```python
from build123d import *

# Parameters (mm, degrees)
F0_W     = 914.4
F0_H     = 914.4
F0_W_2   = 80
F0_H_2   = 40
F1_DEPTH = 40
F2_DEPTH = 1000
F4_W     = 674.4
F4_H     = 40
F5_DEPTH = 127
F7_W     = 674.4
F7_H     = 128
F8_DEPTH = 37
F9_DEPTH = 40


# Not quite as in the source:
# - a feature names something its author has since deleted; it is built from what else it names


with BuildPart() as f1:
    # F0 (on Top) → F1 (new body)
    with BuildSketch(Plane.XY):
        Rectangle(F0_W, F0_H)
        with Locations((-377.2, -407.2)):
            Rectangle(F0_W_2, F0_H_2, mode=Mode.SUBTRACT)
        with Locations((377.2, -407.2)):
            Rectangle(F0_W_2, F0_H_2, mode=Mode.SUBTRACT)
        with Locations((-377.2, 407.2)):
            Rectangle(F0_W_2, F0_H_2, mode=Mode.SUBTRACT)
        with Locations((377.2, 407.2)):
            Rectangle(F0_W_2, F0_H_2, mode=Mode.SUBTRACT)
        with Locations((-377.2, -407.2)):
            Rectangle(F0_W_2, F0_H_2)
        with Locations((377.2, 407.2)):
            Rectangle(F0_W_2, F0_H_2)
        with Locations((377.2, -407.2)):
            Rectangle(F0_W_2, F0_H_2)
        with Locations((-377.2, 407.2)):
            Rectangle(F0_W_2, F0_H_2)
    extrude(amount=F1_DEPTH)

    # F0 (on Top) → F2 (join)
    with BuildSketch(Plane.XY):
        with Locations((-377.2, -407.2)):
            Rectangle(F0_W_2, F0_H_2)
        with Locations((-377.2, 407.2)):
            Rectangle(F0_W_2, F0_H_2)
        with Locations((377.2, -407.2)):
            Rectangle(F0_W_2, F0_H_2)
        with Locations((377.2, 407.2)):
            Rectangle(F0_W_2, F0_H_2)
    extrude(amount=-F2_DEPTH)

    # F4 (on offset) → F5 (join)
    with BuildSketch(Plane.XY.offset(-607)):
        with Locations((0, 407.2)):
            Rectangle(F4_W, F4_H)
    extrude(amount=F5_DEPTH)

    # F7 (on offset) → F8 (join)
    with BuildSketch(Plane.XY.offset(-678)):
        Polygon((-417.2, 387.2), (-417.2, -387.2), (-337.2, -387.2), (-337.2, -64), (-337.2, 64), (-337.2, 387.2), align=None)
        Polygon((337.2, 64), (337.2, -64), (337.2, -387.2), (417.2, -387.2), (417.2, 387.2), (337.2, 387.2), align=None)
        Rectangle(F7_W, F7_H)
    extrude(amount=F8_DEPTH)

    # F9 (cut): a face of the model
    f9_faces = [f1.faces().sort_by_distance(p)[0] for p in [
        (0, 0, 40),
    ]]
    extrude(f9_faces, amount=-F9_DEPTH, mode=Mode.SUBTRACT)


solid = f1.part
```
Check sheet for the modelled part. Datum: model origin and axes. Units: mm. A direction names the side the tool comes from. Coordinates: 2 decimals unless noted, no trailing zeros. Write each loop counter-clockwise with the first axis right and the second up, starting at its lowest first coordinate (ties: lowest second). Pieces come first, ordered by that corner, then holes. Notation, with made-up numbers: M 88,39 L 106,39 A19 cw 106,70 Z; hole C 36,68 d1. An arc over 180 degrees is marked long. Use one line per item in the form item = value.
Item 1: Sectioned sample at C-C, the plane y = 278.5. Record the cut outline in (x, z), and give its area (3 significant figures).
Answer below:
outline = M -417.2,-678 L -337.2,-678 L -337.2,-641 L -417.2,-641 Z; M 337.2,-678 L 417.2,-678 L 417.2,-641 L 337.2,-641 Z
area = 5,920 mm^2
Item 2: Set-up check for faces 4 (the face through (337.2, 312, -672)), 5 (the face through (-5, 407, -607)), 6 (the face through (337.2, 407, -237)), 7 (the face through (-2, 30, -678)), 8 (the face through (-378, -387.2, -316)): record each of +Z, -Z, +X, -X, +Y, -Y from which the full face is reachable in a straight line by a thin tool's end or side.
Answer below:
face_4 = -Z, +Y
face_5 = -Z, +Y, -Y
face_6 = +Z, +Y, -Y
face_7 = -Z, +X, -X
face_8 = +Z, +X, -X
Item 3: Gauge pin test, flat ends, axial feed: pin 1 Ø6 at (x, z) = (-276.5, -655.5) entering from -Y; pin 2 Ø4 at (x, y) = (-60.5, -36.5) entering from +Z. Record the tip position at first contact, or that the pin passes through.
Answer below:
pin_1 = -64
pin_2 = -641
Item 4: Release check for a two-part mould opening along Y. For faces 1 (the face through (-378, -387.2, -837)), 2 (the face through (-337.2, -394, -535)), 3 (the face through (-5, 64, -660)) record: pulls with the +Y half, pulls with the -Y half, needs draft (parallel to the pull), parting line crosses it, or undercut.
Answer below:
face_1 = undercut
face_2 = needs draft
face_3 = pulls with the +Y half
Item 5: Sectioned sample at A-A, the plane z = -886. Record the cut outline in (x, y).
Answer below:
outline = M -417.2,-427.2 L -337.2,-427.2 L -337.2,-387.2 L -417.2,-387.2 Z; M -417.2,387.2 L -337.2,387.2 L -337.2,427.2 L -417.2,427.2 Z; M 337.2,-427.2 L 417.2,-427.2 L 417.2,-387.2 L 337.2,-387.2 Z; M 337.2,387.2 L 417.2,387.2 L 417.2,427.2 L 337.2,427.2 Z
Item 6: Sectioned sample at D-D, the plane y = -47. Record the cut outline in (x, z).
Answer below:
outline = M -417.2,-678 L 417.2,-678 L 417.2,-641 L -417.2,-641 Z
Item 7: Material ranges on L1, parallel to Y at x = -350.5, z = -470; L2, parallel to Z at x = 365, y = -222; L3, parallel to Y at x = 133.5, z = -645, recorded low to high. Write a range as from..to.
Answer below:
L1 = -427.2..-387.2, 387.2..427.2
L2 = -678..-641
L3 = -64..64
Item 8: Sectioned sample at B-B, the plane x = 189.5. Record the cut outline in (y, z).
Answer below:
outline = M -64,-678 L 64,-678 L 64,-641 L -64,-641 Z; M 387.2,-607 L 427.2,-607 L 427.2,-480 L 387.2,-480 Z
